Verification items for this drawing (mm, ordinates from the low corner). A direction names the side the tool comes from. Coordinates: 2 decimals unless noted, no trailing zeros. Order: outer loops, then holes, each group sorted by start corner. A loop starts at its lowest first (then second) coordinate and runs counter-clockwise, first axis right, second up. Notation, with made-up numbers: (67.5, 58) - (89.5, 58) arc R28 ccw to (89.5, 97) - close; hole circle Ø6 at (-8, 16). An arc over 180 degrees is marked (long way). One line per question, with ' | ' between items. Start each with the question number.
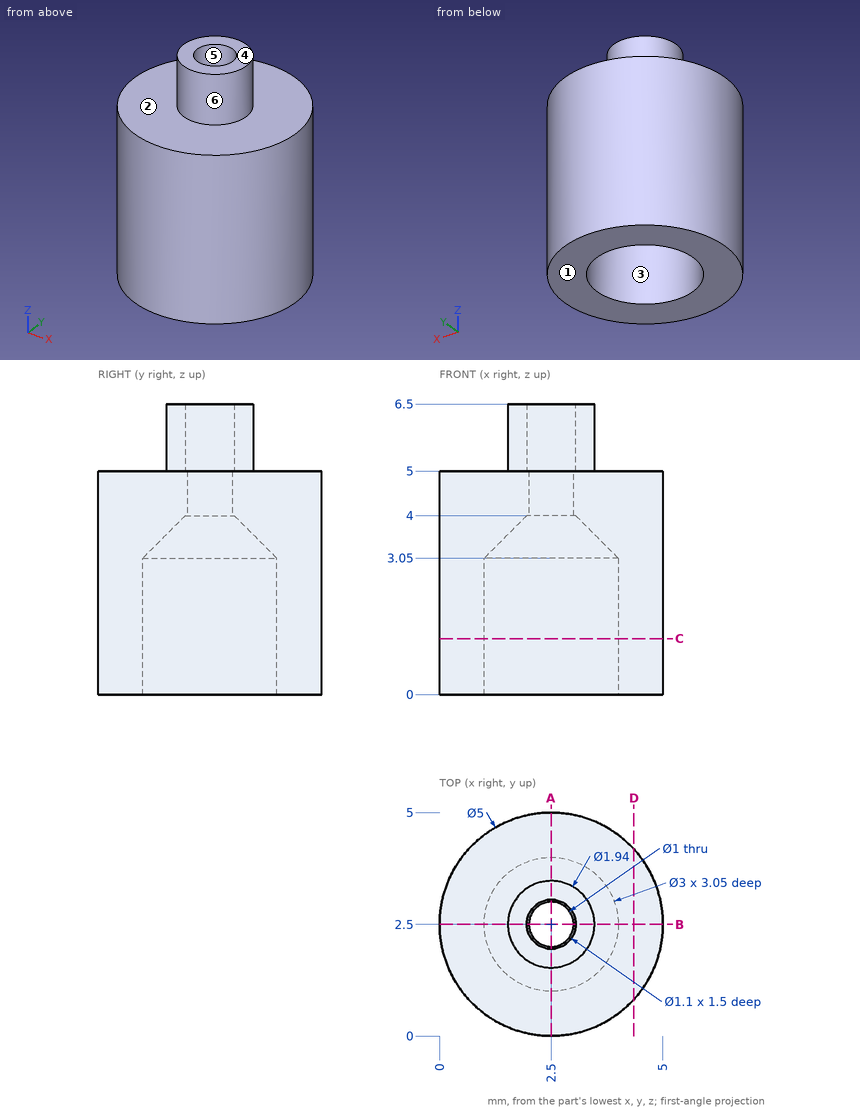
Item 1: Section check D-D (x = 4.35). Record the cut outline in (y, z), then the cut area to 3 significant figures.
Item 2: Mould release check, pull along Y, two halves, no side actions. Record for the marked faces 4, 5 and 6: +Y half, -Y half, draft (parallel to the pull), parting line (faces both ways), or undercut.
Item 3: Gauge pin test, flat ends, axial feed: pin 1 (0.5 mm diameter, centred on x = 2.5, y = 2, fed in from -Z); pin 2 (1 mm diameter, centred on x = 3.5, z = 1, fed in from -Y). Record the tip position at first contact, or that the pin passes through.
Item 4: Set-up check for the marked faces 1, 2 and 3: record each of +Z, -Z, +X, -X, +Y, -Y from which the full face is reachable in a straight line by a thin tool's end or side.
Item 5: Thickness scan on probe 1 along X at (y, z) = (2.5, 1); probe 2 along Y at (x, z) = (2.5, 5.6). Record the ranges inside material, lowest first. Write a range as from..to.
Item 6: Section check C-C (z = 1.25). Record the cut outline in (x, y), then the cut area to 3 significant figures.
Item 7: Section check A-A (x = 2.5). Record the cut outline in (y, z), then the cut area to 3 significant figures.
Completed:
1) outline: (0.82, 0) - (4.18, 0) - (4.18, 5) - (0.82, 5) - close | area: 16.8 mm^2
2) face 4: draft | face 5: undercut | face 6: parting line
3) pin 1: stops at z = 3.8 | pin 2: stops at y = 0.05
4) face 1: -Z, +X, -X, +Y, -Y | face 2: +Z | face 3: -Z
5) probe 1: x = 0..1, 4..5 | probe 2: y = 1.53..1.95, 3.05..3.47
6) outline: circle Ø5 at (2.5, 2.5); hole circle Ø3 at (2.5, 2.5) | area: 12.6 mm^2
7) outline: (0, 0) - (1, 0) - (1, 3.05) - (1.95, 4) - (2, 4) - (2, 5) - (1.95, 5) - (1.95, 6.5) - (1.53, 6.5) - (1.53, 5) - (0, 5) - close; (3, 4) - (3.05, 4) - (4, 3.05) - (4, 0) - (5, 0) - (5, 5) - (3.47, 5) - (3.47, 6.5) - (3.05, 6.5) - (3.05, 5) - (3, 5) - close | area: 14.2 mm^2
